Can you work these out from the model? Positions are in its coordinate system, mm. A direction names the side the tool comes from. Give positions to 0.01 mm unless a question says otherwise; leave off trailing zeros. Write each loop counter-clockwise with the first axis right and the second up, starting at its lowest first coordinate (ties: lowest second). Pieces come first, ordered by that corner, then holes.
from build123d import *

# Parameters (mm, degrees)
SKETCH_1_W          = 53
SKETCH_1_H          = 60
EXTRUDE_1_DEPTH     = 3
EXTRUDE_2_DEPTH     = 22
SKETCH_3_W          = 32
SKETCH_3_H          = 3
EXTRUDE_3_DEPTH     = 50
CUT_EXTRUDE_1_DEPTH = 5
SKETCH_6_W          = 32
SKETCH_6_H          = 3
CUT_EXTRUDE_2_DEPTH = 45
SKETCH_7_R          = 7.5
CUT_EXTRUDE_3_DEPTH = 45
SKETCH_8_R          = 1.75
CUT_EXTRUDE_4_DEPTH = 45
FILLET_1_R          = 3
CHAMFER_1_SIZE      = 2


with BuildPart() as part:
    # 草图1 → 凸台-拉伸1 (new body)
    with BuildSketch(Plane(origin=(0, 0, 0), x_dir=(1, 0, 0), z_dir=(0, 1, 0))):
        with Locations((26.5, 30)):
            Rectangle(SKETCH_1_W, SKETCH_1_H)
    extrude(amount=EXTRUDE_1_DEPTH)

    # 草图2 → 凸台-拉伸2 (add)
    with BuildSketch(Plane(origin=(0, 3, 0), x_dir=(1, 0, 0), z_dir=(0, 1, 0))):
        Polygon((0, 49), (53, 49), (53, 11), (0, 11), (0, 14), (50, 14), (50, 46), (0, 46), align=None)
    extrude(amount=EXTRUDE_2_DEPTH)

    # 草图3 → 凸台-拉伸3 (add)
    with BuildSketch(Plane.ZY.offset(-50)):
        with Locations((-30, 23.5)):
            Rectangle(SKETCH_3_W, SKETCH_3_H)
    extrude(amount=EXTRUDE_3_DEPTH)

    # 草图5 → 切除-拉伸1 (cut)
    with BuildSketch(Plane.ZY):
        Polygon((-49, 25), (-49, 3), (-60, 3), (-60, 0), (0, 0), (0, 3), (-11, 3), (-11, 25), (-14, 25), (-14, 22), (-46, 22), (-46, 25), align=None)
    extrude(amount=-CUT_EXTRUDE_1_DEPTH, mode=Mode.SUBTRACT)

    # 草图6 → 切除-拉伸2 (cut)
    with BuildSketch(Plane.ZY.offset(-5)):
        with Locations((-30, 1.5)):
            Rectangle(SKETCH_6_W, SKETCH_6_H)
    extrude(amount=-CUT_EXTRUDE_2_DEPTH, mode=Mode.SUBTRACT)

    # 草图7 → 切除-拉伸3 (cut)
    with BuildSketch(Plane(origin=(53, 0, 0), x_dir=(0, 0, -1), z_dir=(1, 0, 0))):
        with Locations((30, 12.5)):
            Circle(SKETCH_7_R)
    extrude(amount=-CUT_EXTRUDE_3_DEPTH, mode=Mode.SUBTRACT)

    # 草图8 → 切除-拉伸4 (cut)
    with BuildSketch(Plane.XZ):
        with Locations(Location((10, -5, 0), (0, 0, 270))):
            Circle(SKETCH_8_R)
        with Locations(Location((10, -55, 0), (0, 0, 270))):
            Circle(SKETCH_8_R)
    extrude(amount=-CUT_EXTRUDE_4_DEPTH, mode=Mode.SUBTRACT)

    # 圆角1
    fillet_1_edges = [part.edges().sort_by_distance(p)[0] for p in [
        (0, 23.5, -46),
        (0, 23.5, -14),
        (5, 1.5, 0),
        (5, 1.5, -60),
        (53, 1.5, -60),
        (53, 1.5, 0),
    ]]
    fillet(fillet_1_edges, radius=FILLET_1_R)

    # 倒角1
    chamfer_1_edges = [part.edges().sort_by_distance(p)[0] for p in [
        (5, 23.5, -46),
        (5, 23.5, -14),
    ]]
    chamfer(chamfer_1_edges, length=CHAMFER_1_SIZE - 0.0001)  # a hair under: the kernel refuses the full size


solid = part.part
(1) Imagine slicing it at B-B, the plane z = -55. Write out the boundary of the cut face in (x, y).
Returned:
outline: (5, 0) - (8.25, 0) - (8.25, 3) - (5, 3) - close; (11.75, 0) - (53, 0) - (53, 3) - (11.75, 3) - close
(2) Imagine slicing it at D-D, the plane z = -30. Write out the boundary of the cut face in (x, y), plus the area to 3 significant figures.
Returned:
outline: (0, 22) - (50, 22) - (50, 20) - (53, 20) - (53, 25) - (0, 25) - close; (50, 0) - (53, 0) - (53, 5) - (50, 5) - close
area: 180 mm2
(3) Will these pins go through, and if not, where does the flat tip stop? P1, Ø3.5, axis at x = 37, z = -52, coming from the +Y side; P2, Ø3, axis at x = 45, z = -25, coming from the -Y side; P3, Ø11, axis at y = 14.5, z = -33, coming from the -X side.
Returned:
P1: stops at y = 3
P2: stops at y = 22
P3: stops at x = 50
(4) Imagine slicing it at A-A, the plane y = 17. Write out the boundary of the cut face in (x, z), plus the area to 3 significant figures.
Returned:
outline: (5, -49) - (53, -49) - (53, -36) - (50, -36) - (50, -46) - (5, -46) - close; (5, -14) - (50, -14) - (50, -24) - (53, -24) - (53, -11) - (5, -11) - close
area: 348 mm2
(5) Imagine slicing it at C-C, the plane x = 10. Write out the boundary of the cut face in (y, z).
Returned:
outline: (0, -60) - (3, -60) - (3, -56.75) - (0, -56.75) - close; (0, -53.25) - (3, -53.25) - (3, -49) - (25, -49) - (25, -11) - (3, -11) - (3, -6.75) - (0, -6.75) - (0, -14) - (22, -14) - (22, -46) - (0, -46) - close; (0, -3.25) - (3, -3.25) - (3, 0) - (0, 0) - close
(6) If I drill on L1, parallel to X at y = 1.05, z = -55; L2, parallel to Z at x = 30.5, y = 3.75; L3, parallel to Y at x = 51.5, z = -30, over which ranges is the centre line in solid material (lowest first)?
Returned:
L1: x = 5 to 8.25, 11.75 to 53
L2: z = -49 to -46, -14 to -11
L3: y = 0 to 5, 20 to 25
(7) For faces 4 (the face through (29, 14, -11)), 5 (the face through (50, 4, -30)), 6 (the face through (4, 23, -47)), 7 (the face through (29, 14, -49)), which set-ups out of +Z, -Z, +X, -X, +Y, -Y let a thin tool reach every point of the face, with its end or its side?
Returned:
face 4: +Z, +X, -X, +Y
face 5: -X, -Y
face 6: -Z, -X, +Y, -Y
face 7: -Z, +X, -X, +Y
(8) If we mould it in two halves opening along Z, with no side actions, what happens to faces 1 (the face through (0.9, 23.52, -45.14)), 2 (the face through (27, 11, -14)), 3 (the face through (29, 3, -6))? For each: +Z half, -Z half, draft (parallel to the pull), parting line (faces both ways), or undercut.
Returned:
face 1: -Z half
face 2: undercut
face 3: draft
